Input: part model. Units: mm. Frame: model coordinates. Face numbers are marked on the shaded views. A direction names the side the tool comes from. Round coordinates to 2 decimals unless told otherwise and drop trailing zeros. Loops run counter-clockwise (first coordinate to the right, second up) from the corner with the lowest first, then second, coordinate; pieces in that order, holes last. Notation, with made-up numbers: (58.25, 58.5) -> (74.25, 58.5) arc R25 cw to (74.25, 97.5) -> close; hole circle Ø5 at (67, 57.5). An arc over 180 degrees is marked (long way). One line per question, with ' | ' between items. Start each with the question number.
Q1. Cut plane B-B on z = 82.55. Return loops of the section in (x, y) (3 decimals).
Q2. Access query for the marked faces 1 and 2. Directions: +Z, -Z, +X, -X, +Y, -Y. A direction counts if a zero-diameter tool reaches every point of the face in a straight line with its end or side. Return the directions, or none.
Q3. Material intervals for L1, parallel to Y at x = 4.25, z = 39 (3 decimals); L2, parallel to X at y = 17, z = 23.5 (3 decimals); L3, parallel to X at y = 40.25, z = 19.05, sorted ascending.
Q4. Cut plane C-C on z = 49. Return loops of the section in (x, y) (3 decimals).
Q5. Cut plane A-A on x = 12.7. State how many separate pieces and enclosed holes the cut face has, and give its area (3 significant figures).
Q6. Cut plane D-D on y = 17.5. Return loops of the section in (x, z) (3 decimals).
Q7. Contact query for flat-ended pins moving along their axis: P1, Ø6, axis at x = 14, z = 54, coming from the -Y side; P2, Ø3, axis at x = 12.7, z = 82.55, coming from the -Y side; P3, Ø18.5, axis at y = 24.5, z = 49.5, coming from the +X side. Output: stop coordinate, or through.
from build123d import *

# Parameters (mm, degrees)
BASE_FLANGE1_DEPTH         = 88.9
F_8_0_199_DIAMETER_HOLE1_D = 5.0546


# Sheet-metal steps are written as plain solids
with BuildPart() as part:
    # Sketch1 → Base-Flange1 (new body)
    with BuildSketch(Plane.XY):
        with BuildLine():
            Line((0, 0), (0, 36.576))
            ThreePointArc((0, 36.576), (0.446369265, 37.653630735), (1.524, 38.1))
            Line((1.524, 38.1), (16.51, 38.1))
            Line((16.51, 38.1), (16.51, 41.275))
            Line((16.51, 41.275), (1.524, 41.275))
            ThreePointArc((1.524, 41.275), (-1.798694765, 39.898694765), (-3.175, 36.576))
            Line((-3.175, 36.576), (-3.175, 0))
            Line((-3.175, 0), (0, 0))
        make_face()
    extrude(amount=BASE_FLANGE1_DEPTH)

    # #8 (0.199) Diameter Hole1 (through all)
    with Locations(Plane(origin=(12.7, 41.275, 6.35), x_dir=(0, 0, 1), z_dir=(0, 1, 0))):
        with Locations((0, 0), (12.7, 0), (25.4, 0), (38.1, 0), (50.8, 0), (63.5, 0), (76.2, 0)):
            Hole(F_8_0_199_DIAMETER_HOLE1_D / 2)


solid = part.part
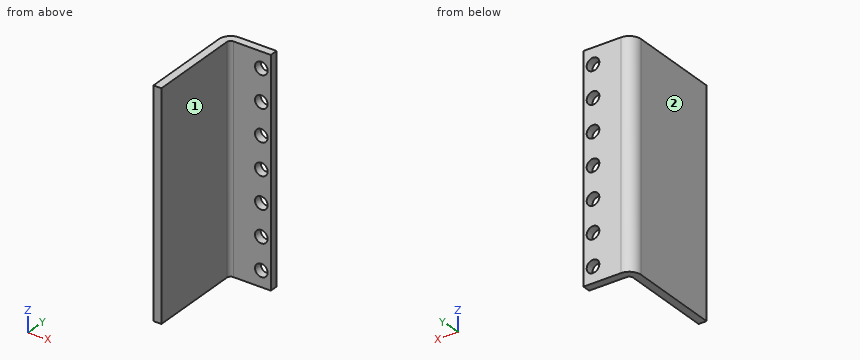
Results:
1) outline: (-3.175, 0) -> (0, 0) -> (0, 36.576) arc R1.524 cw to (1.524, 38.1) -> (10.173, 38.1) -> (10.173, 41.275) -> (1.524, 41.275) arc R4.699 ccw to (-3.175, 36.576) -> close; (15.227, 38.1) -> (16.51, 38.1) -> (16.51, 41.275) -> (15.227, 41.275) -> close
2) face 1: +Z, -Z, +X, -Y | face 2: +Z, -Z, -X, +Y, -Y
3) L1: 38.1 to 41.275 | L2: -3.175 to 0 | L3: -1.41 to 10.17, 15.23 to 16.51
4) outline: (-3.175, 0) -> (0, 0) -> (0, 36.576) arc R1.524 cw to (1.524, 38.1) -> (16.51, 38.1) -> (16.51, 41.275) -> (1.524, 41.275) arc R4.699 ccw to (-3.175, 36.576) -> close
5) separate pieces: 8 | enclosed holes: 0 | area: 170 mm^2
6) outline: (-3.175, 0) -> (0, 0) -> (0, 88.9) -> (-3.175, 88.9) -> close
7) P1: y = 38.1 | P2: through | P3: x = 0
